Can you work these out from the model? Positions are in its coordinate system, mm. Face numbers are marked on the shaded views. A direction names the side the tool comes from. Give positions to 0.01 mm unless a question says otherwise; leave off trailing zeros. Write each loop counter-clockwise with the first axis right and the second up, starting at its lowest first coordinate (ties: lowest second). Pieces come first, ordered by that corner, then holes. Notation, with made-up numbers: M -3.75,45.5 L 26.25,45.5 A18 ccw 26.25,64.5 Z; hole C -1.75,-38 d9. An arc over 180 degrees is marked long. Write each question's results on one line, items separated by ' | '.
from build123d import *

# Parameters (mm, degrees)
SKETCH2_W                      = 9.525
SKETCH2_H                      = 4.75615
CUT_EXTRUDE1_REACH             = 69.93
SKETCH4_W                      = 9.525
SKETCH4_H                      = 7.14375
CUT_EXTRUDE1_DIRECTION_2_DEPTH = 68.929971613
FILLET1_R                      = 0.381
CUT_EXTRUDE2_DEPTH             = 71.918317263
CUT_EXTRUDE2_DEPTH_BACK        = 71.918317263
F_3_16_0_1875_DIAMETER_HOLE1_D = 4.7625


with BuildPart() as part:
    # Sketch1 → Revolve1 (revolve)
    with BuildSketch(Plane.XY):
        Polygon((-43.65625, 0), (-43.65625, 4.7625), (0, 4.7625), (0, 6.5484375), (2.159, 6.5484375), (2.159, 19.05), (7.2898, 19.05), (7.2898, 0), align=None)
        Polygon((16.8148, 4.7625), (16.8148, 19.05), (21.9456, 19.05), (21.9456, 7.9375), (24.1046, 7.9375), (24.1046, 6.35), (43.94835, 6.35), (43.94835, 4.7625), align=None)
    revolve(axis=Axis((0, 0, 0), (-1, 0, 0)))

    # Sketch2 → Revolve2 (revolve)
    with BuildSketch(Plane.XY, mode=Mode.PRIVATE) as revolve2_sk:
        with Locations((12.0523, 15.078075)):
            Rectangle(SKETCH2_W, SKETCH2_H)
    revolve(revolve2_sk.sketch.rotate(Axis((-15.553486907, 12.7, 0), (1, 0, 0)), 90), axis=Axis((-15.553486907, 12.7, 0), (1, 0, 0)))

    # Sketch4 → Cut-Extrude1 (cut, up to next)
    with BuildSketch(Plane(origin=(7.2898, 6.51548373, -17.901144426), x_dir=(-1, 0, 0), z_dir=(0, 0.34202014332566627, -0.9396926207859093)), mode=Mode.PRIVATE) as cut_extrude1_sk1:
        with Locations((-29.911675, 0)):
            Rectangle(SKETCH4_W, SKETCH4_H)
    cut_extrude1_tool1 = extrude(cut_extrude1_sk1.sketch, amount=-CUT_EXTRUDE1_REACH, mode=Mode.PRIVATE) & part.part
    add(cut_extrude1_tool1.solids().sort_by_distance((37.201475, 6.515484, -17.901144))[0], mode=Mode.SUBTRACT)

    # Sketch4 → Cut-Extrude1 direction 2 (cut)
    with BuildSketch(Plane(origin=(7.2898, 6.51548373, -17.901144426), x_dir=(-1, 0, 0), z_dir=(0, 0.34202014332566627, -0.9396926207859093))):
        with Locations((-29.911675, 0)):
            Rectangle(SKETCH4_W, SKETCH4_H)
    extrude(amount=CUT_EXTRUDE1_DIRECTION_2_DEPTH, mode=Mode.SUBTRACT)

    # Fillet1
    fillet1_edges = [part.edges().sort_by_distance(p)[0] for p in [
        (7.2898, 12.7, -4.75615),
        (16.8148, 12.7, -4.75615),
    ]]
    fillet(fillet1_edges, radius=FILLET1_R)

    # Sketch5 → Cut-Extrude2 (cut, two sides: drawn at the far end of the back side and taken through both)
    with BuildSketch(Plane(origin=(21.9456, 0, 0), x_dir=(0, 0, -1), z_dir=(1, 0, 0)).offset(-CUT_EXTRUDE2_DEPTH_BACK)):
        with BuildLine():
            ThreePointArc((-6.291289262, 13.561498357), (-4.174445198, 17.485029497), (2e-09, 19.05))
            ThreePointArc((2e-09, 19.05), (-13.470384181, 13.470384182), (-19.05, 0))
            Line((-19.05, 0), (-12.303125, 0))
            ThreePointArc((-12.303125, 0), (-9.172291101, 1.173727878), (-7.584658053, 4.116376233))
            Line((-7.584658053, 4.116376233), (-6.291289262, 13.561498357))
        make_face()
        with BuildLine():
            ThreePointArc((7.584658053, 4.116376233), (9.172291101, 1.173727878), (12.303125, 0))
            Line((12.303125, 0), (19.05, 0))
            ThreePointArc((19.05, 0), (13.470384182, 13.470384181), (2e-09, 19.05))
            ThreePointArc((2e-09, 19.05), (4.1744452, 17.485029496), (6.291289262, 13.561498357))
            Line((6.291289262, 13.561498357), (7.584658053, 4.116376233))
        make_face()
    extrude(amount=CUT_EXTRUDE2_DEPTH + CUT_EXTRUDE2_DEPTH_BACK, mode=Mode.SUBTRACT)

    # 3/16 (0.1875) Diameter Hole1 (through all)
    with Locations(Plane.ZY.offset(-2.159)):
        with Locations((0, 12.7)):
            Hole(F_3_16_0_1875_DIAMETER_HOLE1_D / 2)


solid = part.part
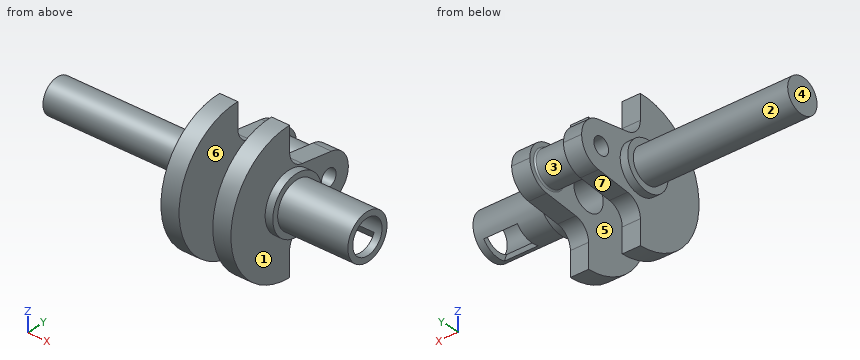
Item 1: I want a section at C-C, the plane y = 2. Give the number of separate pieces and of enclosed holes in the cut face, and give its area (3 significant figures).
Geometry says:
separate pieces: 4 | enclosed holes: 0 | area: 599 mm2
Item 2: If I drill on line 1 (X direction, y = 4.5, z = -3.5); line 2 (Z direction, x = 25.75, y = 0); line 3 (X direction, y = 8, z = 3), over which ranges is the centre line in solid material (lowest first)? Write a range as from..to.
Geometry says:
line 1: x = 0..7.29, 16.81..32.44, 41.96..43.95 | line 2: z = -6.35..-4.76, 4.76..6.35 | line 3: x = 2.16..7.29, 16.81..21.95
Item 3: I want a section at A-A, the plane y = -10.5. Please give me the cut outline in (x, z).
Geometry says:
outline: M 2.16,-15.9 L 7.29,-15.9 L 7.29,15.9 L 2.16,15.9 Z; M 16.81,-15.9 L 21.95,-15.9 L 21.95,15.9 L 16.81,15.9 Z
Item 4: Thinking about a two-plate mould opening in X: for the marked faces 4, 5, 6 and 7, which applies, +X half, -X half, draft (parallel to the pull), parting line (faces both ways), or undercut?
Geometry says:
face 4: -X half | face 5: undercut | face 6: undercut | face 7: draft
Item 5: I'm going to push flat-ended pins straight in: pin 1 (5.5 mm diameter, centred on x = 3.5, z = 17, fed in from +Y); pin 2 (1.4 mm diameter, centred on y = 2, z = -3.5, fed in from +X); pin 3 (4 mm diameter, centred on x = 2.5, y = -11.5, fed in from -Z). Where does each tip first touch, or does it pass through?
Geometry says:
pin 1: stops at y = 0 | pin 2: stops at x = 7.29 | pin 3: stops at z = -16.51
Item 6: I want a section at B-B, the plane z = -17. Please give me the cut outline in (x, y).
Geometry says:
outline: M 2.16,-8.6 L 7.29,-8.6 L 7.29,0 L 2.16,0 Z; M 16.81,-8.6 L 21.95,-8.6 L 21.95,0 L 16.81,0 Z
Item 7: For the marked faces 1, 2 and 3, which set-ups out of +Z, -Z, +X, -X, +Y, -Y let a thin tool reach every point of the face, with its end or its side?
Geometry says:
face 1: +X | face 2: -X | face 3: none
